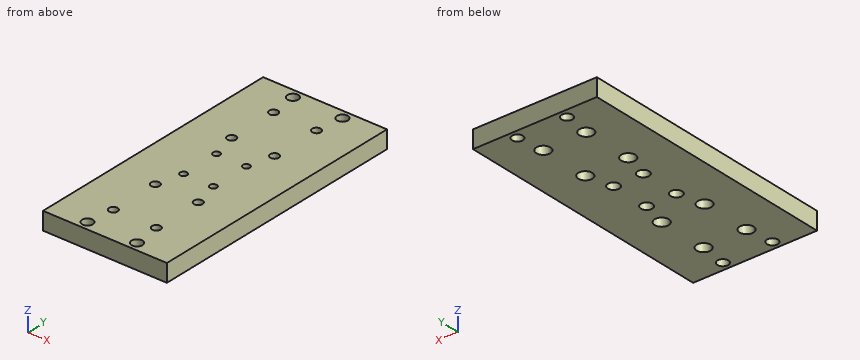
```python
from build123d import *

# Parameters (mm, degrees)
ESBO_O1_W                                   = 75
ESBO_O1_H                                   = 160
RESSALTO_EXTRUS_O1_DEPTH                    = 10.7
FURO_ROSCADO_PARA_CONDU_TE_DE_1_4_281_D     = 6.6294
FURO_ROSCADO_PARA_CONDU_TE_DE_1_4_281_DEPTH = 15
FURO_ROSCADO_PARA_CONDU_TE_DE_1_4_281_TIP   = 1.991672694
FURO_ROSCADO_PARA_CONDU_TE_DE_M5X0_81_D     = 5.2
FURO_ROSCADO_PARA_CONDU_TE_DE_M5X0_81_DEPTH = 15
FURO_ROSCADO_PARA_CONDU_TE_DE_M5X0_81_TIP   = 1.562237609
FURO_ROSCADO_PARA_CONDU_TE_DE_M4X0_71_D     = 4.2
FURO_ROSCADO_PARA_CONDU_TE_DE_M4X0_71_DEPTH = 15
FURO_ROSCADO_PARA_CONDU_TE_DE_M4X0_71_TIP   = 1.2618073
ESBO_O8_R                                   = 4.25
CORTE_EXTRUS_O1_DEPTH                       = 5
ESBO_O9_R                                   = 3.5
CORTE_EXTRUS_O2_DEPTH                       = 4


with BuildPart() as part:
    # Esboço1 → Ressalto-extrusão1 (new body)
    with BuildSketch(Plane.XY):
        Rectangle(ESBO_O1_W, ESBO_O1_H)
    extrude(amount=RESSALTO_EXTRUS_O1_DEPTH)

    # Furo roscado para conduíte de 1/4-281
    with Locations(Plane(origin=(0, 0, 0), x_dir=(-1, 0, 0), z_dir=(0, 0, -1))):
        with Locations((15, 74.65), (-15, 74.65), (15, -74.65), (-15, -74.65)):
            Hole(FURO_ROSCADO_PARA_CONDU_TE_DE_1_4_281_D / 2, depth=FURO_ROSCADO_PARA_CONDU_TE_DE_1_4_281_DEPTH)
            with Locations((0, 0, -(FURO_ROSCADO_PARA_CONDU_TE_DE_1_4_281_DEPTH + FURO_ROSCADO_PARA_CONDU_TE_DE_1_4_281_TIP / 2))):  # 118° drill point
                Cone(0, FURO_ROSCADO_PARA_CONDU_TE_DE_1_4_281_D / 2, FURO_ROSCADO_PARA_CONDU_TE_DE_1_4_281_TIP, mode=Mode.SUBTRACT)

    # Furo roscado para conduíte de M5x0.81
    with Locations(Plane(origin=(0, 0, 0), x_dir=(-1, 0, 0), z_dir=(0, 0, -1))):
        with Locations((13, 58.25), (13, 27.75), (-13, 27.75), (-13, 58.25), (13, -27.75), (-13, -27.75), (13, -58.25), (-13, -58.25)):
            Hole(FURO_ROSCADO_PARA_CONDU_TE_DE_M5X0_81_D / 2, depth=FURO_ROSCADO_PARA_CONDU_TE_DE_M5X0_81_DEPTH)
            with Locations((0, 0, -(FURO_ROSCADO_PARA_CONDU_TE_DE_M5X0_81_DEPTH + FURO_ROSCADO_PARA_CONDU_TE_DE_M5X0_81_TIP / 2))):  # 118° drill point
                Cone(0, FURO_ROSCADO_PARA_CONDU_TE_DE_M5X0_81_D / 2, FURO_ROSCADO_PARA_CONDU_TE_DE_M5X0_81_TIP, mode=Mode.SUBTRACT)

    # Furo roscado para conduíte de M4x0.71
    with Locations(Plane(origin=(0, 0, 0), x_dir=(-1, 0, 0), z_dir=(0, 0, -1))):
        with Locations((9, 12), (-9, 12), (9, -12), (-9, -12)):
            Hole(FURO_ROSCADO_PARA_CONDU_TE_DE_M4X0_71_D / 2, depth=FURO_ROSCADO_PARA_CONDU_TE_DE_M4X0_71_DEPTH)
            with Locations((0, 0, -(FURO_ROSCADO_PARA_CONDU_TE_DE_M4X0_71_DEPTH + FURO_ROSCADO_PARA_CONDU_TE_DE_M4X0_71_TIP / 2))):  # 118° drill point
                Cone(0, FURO_ROSCADO_PARA_CONDU_TE_DE_M4X0_71_D / 2, FURO_ROSCADO_PARA_CONDU_TE_DE_M4X0_71_TIP, mode=Mode.SUBTRACT)

    # Esboço8 → Corte-extrusão1 (cut)
    with BuildSketch(Plane(origin=(0, 0, 0), x_dir=(-1, 0, 0), z_dir=(0, 0, -1))):
        with Locations((-13, 58.25)):
            Circle(ESBO_O8_R)
        with Locations((-13, 27.75)):
            Circle(ESBO_O8_R)
        with Locations((13, 27.75)):
            Circle(ESBO_O8_R)
        with Locations((13, 58.25)):
            Circle(ESBO_O8_R)
        with Locations((13, -27.75)):
            Circle(ESBO_O8_R)
        with Locations((-13, -27.75)):
            Circle(ESBO_O8_R)
        with Locations((13, -58.25)):
            Circle(ESBO_O8_R)
        with Locations((-13, -58.25)):
            Circle(ESBO_O8_R)
    extrude(amount=-CORTE_EXTRUS_O1_DEPTH, mode=Mode.SUBTRACT)

    # Esboço9 → Corte-extrusão2 (cut)
    with BuildSketch(Plane(origin=(0, 0, 0), x_dir=(-1, 0, 0), z_dir=(0, 0, -1))):
        with Locations((-9, 12)):
            Circle(ESBO_O9_R)
        with Locations((9, 12)):
            Circle(ESBO_O9_R)
        with Locations((-9, -12)):
            Circle(ESBO_O9_R)
        with Locations((9, -12)):
            Circle(ESBO_O9_R)
    extrude(amount=-CORTE_EXTRUS_O2_DEPTH, mode=Mode.SUBTRACT)


solid = part.part
```
Read the model definition and answer for the solid it produces. Units are mm, in the model's axes. Round coordinates to 2 decimals unless told otherwise and drop trailing zeros. Write each loop counter-clockwise with the first axis right and the second up, starting at its lowest first coordinate (ties: lowest second). Pieces come first, ordered by that corner, then holes. Notation, with made-up numbers: (19.5, 55) - (28.5, 55) arc R37 ccw to (28.5, 94) - close; hole circle Ø1 at (59.5, -36). An arc over 180 degrees is marked (long way). Use CSV: the item, a comma, the result in double quotes.
Q1. Find section C-C, the plane y = -27.75. Write down the section's boundary in (x, z).
Values:
outline,"(-37.5, 0) - (-17.25, 0) - (-17.25, 5) - (-15.6, 5) - (-15.6, 10.7) - (-37.5, 10.7) - close; (-10.4, 5) - (-8.75, 5) - (-8.75, 0) - (8.75, 0) - (8.75, 5) - (10.4, 5) - (10.4, 10.7) - (-10.4, 10.7) - close; (15.6, 5) - (17.25, 5) - (17.25, 0) - (37.5, 0) - (37.5, 10.7) - (15.6, 10.7) - close"
Q2. This flat-tipped pin is pushed along its axis until it touches: pin 1 Ø7.5 at (x, y) = (13, -58.25) entering from -Z. Where does it stop, or does it pass through?
Values:
pin 1,"stops at z = 5"
Q3. Find section A-A, the plane y = 74.65. Write down the section's boundary in (x, z), then the cut area to 3 significant figures.
Values:
outline,"(-37.5, 0) - (-18.31, 0) - (-18.31, 10.7) - (-37.5, 10.7) - close; (-11.69, 0) - (11.69, 0) - (11.69, 10.7) - (-11.69, 10.7) - close; (18.31, 0) - (37.5, 0) - (37.5, 10.7) - (18.31, 10.7) - close"
area,"661 mm²"
Q4. Find section B-B, the plane z = 7.25. Count the separate pieces of the cut face and the enclosed holes in it, then the cut area to 3 significant figures.
Values:
separate pieces,"1"
enclosed holes,"16"
area,"11,600 mm²"
Q5. Straight lines are drawn through the part: line 1 along Y through (x, z) = (7.5, 4.5); line 2 along X through (y, z) = (11, 5.75); line 3 along Y through (x, z) = (-7, 2.25). For each, find the intervals that lie inside material, in ascending order.
Values:
line 1,"y = -80 to -13.47, -10.53 to 10.53, 13.47 to 80"
line 2,"x = -37.5 to -10.85, -7.15 to 7.15, 10.85 to 37.5"
line 3,"y = -80 to -14.87, -9.13 to 9.13, 14.87 to 80"
